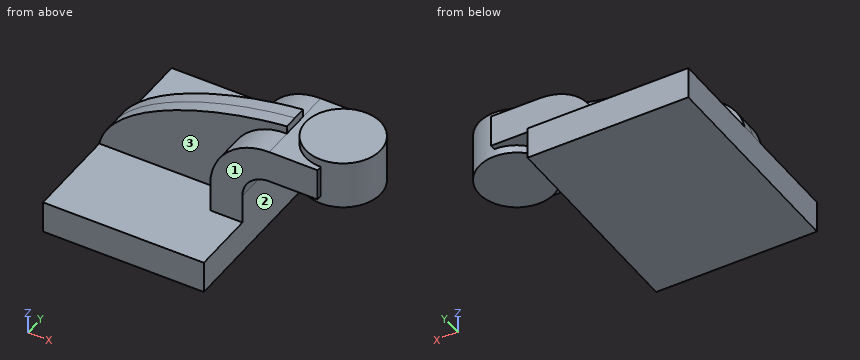
```python
from build123d import *

# Parameters (mm, degrees)
F1_DEPTH = 63.5
F0_W     = 28.575
F0_H     = 19.05
F2_DEPTH = 25.4
F3_DEPTH = 7.9375


with BuildPart() as f1:
    # F0 (on Front) → F1 (new body, symmetric)
    with BuildSketch(Plane.XZ):
        Polygon((-47.625, 9.525), (-47.625, -9.525), (47.625, -9.525), (47.625, 9.525), (28.575, 9.525), align=None)
    extrude(amount=F1_DEPTH, both=True)

    # F0 (on Front) → F2 (join, symmetric)
    with BuildSketch(Plane.XZ):
        with BuildLine():
            Line((28.575, 9.525), (47.625, 9.525))
            Line((47.625, 9.525), (47.625, 27.0002))
            ThreePointArc((47.625, 27.0002), (52.27468, 38.22552), (63.5, 42.8752))
            Line((63.5, 42.8752), (63.5, 61.9252))
            ThreePointArc((63.5, 61.9252), (38.804296, 51.695904), (28.575, 27.0002))
            Line((28.575, 27.0002), (28.575, 9.525))
        make_face()
        with Locations((77.7875, 52.4002)):
            Rectangle(F0_W, F0_H)
    extrude(amount=F2_DEPTH, both=True)

    # F0 (on Front) → F3 (join, symmetric)
    with BuildSketch(Plane.XZ):
        with BuildLine():
            add(Edge.make_bspline(
                [(-47.625, 9.525), (-41.878503, 39.32336), (13.729675, 61.214211), (63.5, 66.675)],
                knots=[0, 0, 0, 0, 124.959546, 124.959546, 124.959546, 124.959546], degree=3))
            Line((-47.625, 9.525), (28.575, 9.525))
            Line((28.575, 9.525), (28.575, 27.0002))
            ThreePointArc((28.575, 27.0002), (38.804296, 51.695904), (63.5, 61.9252))
            Line((63.5, 61.9252), (63.5, 66.675))
        make_face()
    extrude(amount=F3_DEPTH, both=True)

    # F0 (on Front) → F4 (revolve)
    with BuildSketch(Plane.XZ):
        Polygon((114.3, 66.675), (92.075, 66.675), (92.075, 61.9252), (92.075, 42.8752), (92.075, 38.1), (114.3, 38.1), align=None)
    revolve(axis=Axis((92.075, 0, 52.3875), (0, 0, 1)))


solid = f1.part
```
The model under review builds one solid part; all positions refer to its coordinate system, in mm. Face numbers are marked on the shaded views. A direction names the side the tool comes from. Round coordinates to 2 decimals unless told otherwise and drop trailing zeros. Loops run counter-clockwise (first coordinate to the right, second up) from the corner with the lowest first, then second, coordinate; pieces in that order, holes last. Notation, with made-up numbers: (-0.5, 18.25) -> (33.5, 18.25) arc R30 ccw to (33.5, 57.25) -> close; hole circle Ø1 at (-31, 31). An arc over 180 degrees is marked (long way). Answer as a JSON object with one key per item and string values. Group by question number.
1) We need section B-B on y = 54.5. Write out the cut boundary in (x, z) (3 decimals).
2) We need section A-A on z = 3. Write out the cut boundary in (x, y) (3 decimals), then the cut area to 3 significant figures.
3) For the marked faces 1, 2 and 3, list the 3-axis set-ups (+Z, -Z, +X, -X, +Y, -Y) from which the entire face can be reached by the end or side of a thin tool; tool diameter is ignored.
4) For line 1 (Y direction, x = 18, z = 55.5); line 2 (Z direction, x = -29, y = -22) (3 decimals); line 3 (Z direction, x = 70, y = 24), list the stretches that pass through material, from the lowest coordinate up. Write a range as [from, to].
5) We need section C-C on x = 80.5. Write out the cut boundary in (y, z) (3 decimals), then the cut area to 3 significant figures.
6) For pin 1 Ø10 at (x, z) = (-13, 33.5) entering from +Y; pin 2 Ø1 at (y, z) = (-2.5, 13.5) entering from -X; pin 3 Ø6 at (x, y) = (63.5, 13) entering from -Z; pin 4 Ø6 at (x, z) = (-31, 39) entering from -Y, all flat-tipped, find the tip position at first contact; note any pin that passes through.
Result set:
{
 "1": {"outline": "(-47.625, -9.525) -> (47.625, -9.525) -> (47.625, 9.525) -> (-47.625, 9.525) -> close"},
 "2": {"outline": "(-47.625, -63.5) -> (47.625, -63.5) -> (47.625, 63.5) -> (-47.625, 63.5) -> close", "area": "12,100 mm²"},
 "3": {"face 1": "+Z, +X, -X, -Y", "face 2": "-Z, +X, +Y, -Y", "face 3": "+Z, -X, -Y"},
 "4": {"line 1": "[-7.94, 7.94]", "line 2": "[-9.525, 9.525]", "line 3": "[42.88, 61.93]"},
 "5": {"outline": "(-25.4, 42.875) -> (-18.973, 42.875) -> (-18.973, 38.1) -> (18.973, 38.1) -> (18.973, 42.875) -> (25.4, 42.875) -> (25.4, 61.925) -> (18.973, 61.925) -> (18.973, 66.675) -> (-18.973, 66.675) -> (-18.973, 61.925) -> (-25.4, 61.925) -> close", "area": "1,330 mm²"},
 "6": {"pin 1": "y = 7.94", "pin 2": "x = -46.72", "pin 3": "z = 42.59", "pin 4": "through"}
}
